```python
from build123d import *

# Parameters (mm, degrees)
F0_W     = 64
F0_H     = 15
F1_DEPTH = 15
F2_R     = 2.5
F3_DEPTH = 64.001
F4_W     = 4
F4_H     = 8
F5_DEPTH = 11.5
F6_W     = 1
F6_H     = 8
F7_DEPTH = 1


with BuildPart() as f1:
    # F0 (on Top) → F1 (new body)
    with BuildSketch(Plane.XY):
        with Locations((32, 7.5)):
            Rectangle(F0_W, F0_H)
    extrude(amount=F1_DEPTH)

    # F2 (on face) → F3 (cut, through all)
    with BuildSketch(Plane.YZ.offset(64)):
        with Locations((7.5, 7.5)):
            Circle(F2_R)
    extrude(amount=-F3_DEPTH, mode=Mode.SUBTRACT)

    # F4 (on face) → F5 (cut)
    with BuildSketch(Plane.XY.offset(15)):
        with Locations((12, 7.5)):
            Rectangle(F4_W, F4_H)
        with Locations((52, 7.5)):
            Rectangle(F4_W, F4_H)
    extrude(amount=-F5_DEPTH, mode=Mode.SUBTRACT)

    # F6 (on face) → F7 (join)
    with BuildSketch(Plane.XY.offset(15)):
        with Locations((13.5, 7.5)):
            Rectangle(F6_W, F6_H)
        with Locations((50.5, 7.5)):
            Rectangle(F6_W, F6_H)
    extrude(amount=-F7_DEPTH)


solid = f1.part
```
Input: part model. Units: mm. Frame: model coordinates. A direction names the side the tool comes from. Round coordinates to 2 decimals unless told otherwise and drop trailing zeros. Order: outer loops, then holes, each group sorted by start corner. A loop starts at its lowest first (then second) coordinate and runs counter-clockwise, first axis right, second up. Notation, with made-up numbers: (-21, 33.5) - (2, 33.5) arc R29 ccw to (2, 57.5) - close; hole circle Ø3 at (-26, 19.5). An arc over 180 degrees is marked (long way). One line per question, with ' | ' between items. Start each with the question number.
1) Cut plane B-B, the plane y = 7.5. Return the cut outline in (x, z).
2) Set-up query: faces 1 (the flat face through (54, 7, 11)), 2 (the flat face through (12, 8, 3.5)), 3 (the cylindrical face through (5.07, 8.65, 5.28)). Return all of +Z, -Z, +X, -X, +Y, -Y with unobstructed straight access to the full face (end or side cutting, diameter ignored); none if empty.
3) Pull-direction query (Z, two-part tool) for faces 4 (the flat face through (52, 3.5, 9)), 5 (the flat face through (32, 8, 15)), 6 (the flat face through (0, 4, 7)), 7 (the flat face through (32, 8, 0)); classes: +Z half, -Z half, draft (parallel to the pull), parting line (faces both ways), or undercut.
4) Ray query, probe 1 along X at (y, z) = (4, 6.75); probe 2 along Z at (x, y) = (5.25, 7.5); probe 3 along Y at (x, z) = (51.5, 10). Return the intervals inside material, ascending.
5) Cut plane C-C, the plane z = 11. Return the cut outline in (x, y).
6) Cut plane D-D, the plane x = 38. Return the cut outline in (y, z).
7) Cut plane A-A, the plane z = 7.5. Return the cut outline in (x, y), then the cut area to 3 significant figures.
Worked out:
1) outline: (0, 0) - (64, 0) - (64, 5) - (54, 5) - (54, 3.5) - (50, 3.5) - (50, 5) - (14, 5) - (14, 3.5) - (10, 3.5) - (10, 5) - (0, 5) - close; (0, 10) - (10, 10) - (10, 15) - (0, 15) - close; (13, 14) - (14, 14) - (14, 10) - (50, 10) - (50, 14) - (51, 14) - (51, 15) - (13, 15) - close; (54, 10) - (64, 10) - (64, 15) - (54, 15) - close
2) face 1: +Z | face 2: none | face 3: +X, -X
3) face 4: undercut | face 5: +Z half | face 6: draft | face 7: -Z half
4) probe 1: x = 0 to 10, 14 to 50, 54 to 64 | probe 2: z = 0 to 5, 10 to 15 | probe 3: y = 0 to 3.5, 11.5 to 15
5) outline: (0, 0) - (64, 0) - (64, 15) - (0, 15) - close; hole (10, 3.5) - (14, 3.5) - (14, 11.5) - (10, 11.5) - close; hole (50, 3.5) - (54, 3.5) - (54, 11.5) - (50, 11.5) - close
6) outline: (0, 0) - (15, 0) - (15, 15) - (0, 15) - close; hole circle Ø5 at (7.5, 7.5)
7) outline: (0, 0) - (64, 0) - (64, 5) - (54, 5) - (54, 3.5) - (50, 3.5) - (50, 5) - (14, 5) - (14, 3.5) - (10, 3.5) - (10, 5) - (0, 5) - close; (0, 10) - (10, 10) - (10, 11.5) - (14, 11.5) - (14, 10) - (50, 10) - (50, 11.5) - (54, 11.5) - (54, 10) - (64, 10) - (64, 15) - (0, 15) - close | area: 616 mm^2
